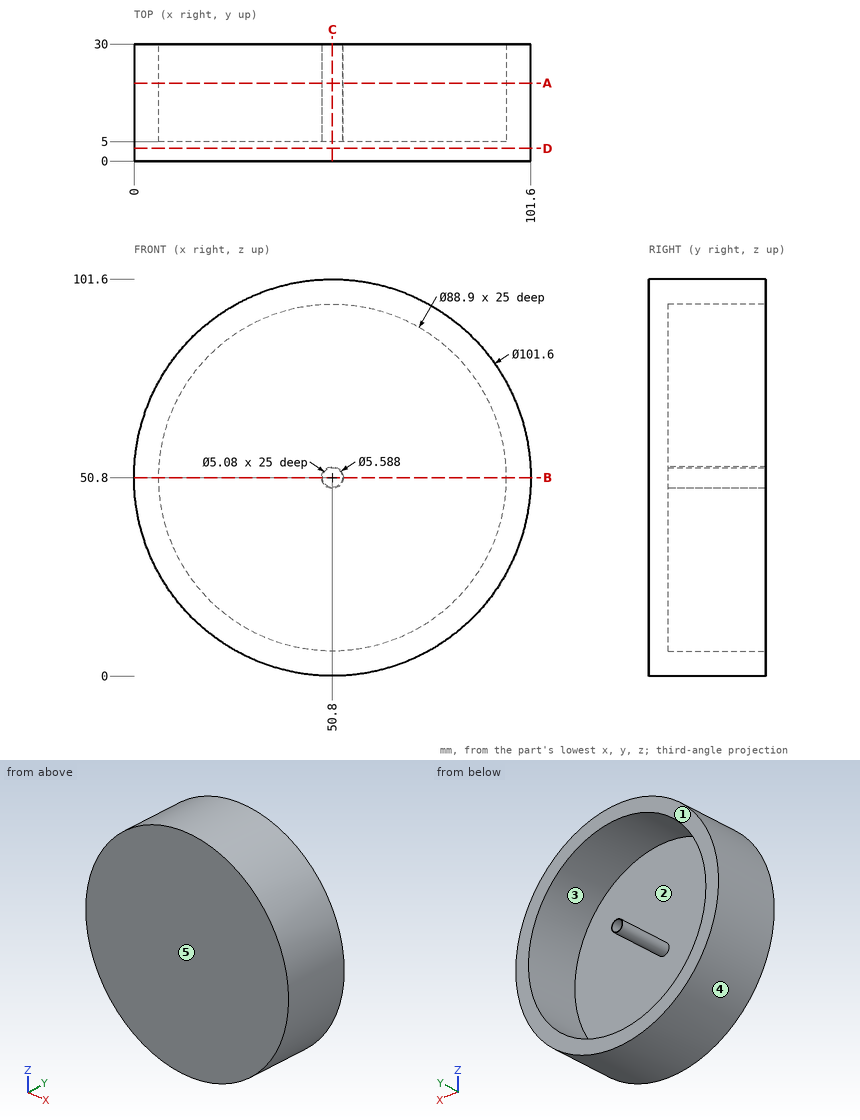
For this review, use the dimensioned drawing (mm, ordinates from the lowest corner) and the shaded views. A direction names the side the tool comes from. Round coordinates to 2 decimals unless told otherwise and drop trailing zeros. Order: outer loops, then holes, each group sorted by start corner. A loop starts at its lowest first (then second) coordinate and runs counter-clockwise, first axis right, second up. Notation, with made-up numbers: (83.25, 61) -> (118.25, 61) arc R19 cw to (118.25, 96) -> close; hole circle Ø8 at (-2, 26.25). An arc over 180 degrees is marked (long way). One line per item, written item: value. Start each with the question number.
Q1. Wall thickness on line 1 (Z direction, x = 50.8, y = 23.5); line 2 (Z direction, x = 55, y = 15.75): over which ranges is each line inside the solid? List them lowest first.
Q2. Mouldability with a two-part tool opening along X and no side actions: class the marked faces 3, 4 and 5 as released by +X, released by -X, zero draft, split by the parting line, or undercut.
Q3. Machinability: for the marked faces 1 and 2, which of the approach directions +Z, -Z, +X, -X, +Y, -Y give a long, thin tool a straight path to every point of the face, cutting with its end or side? Answer none if there is none.
Q4. Take a section at B-B (z = 50.8). Write out the cut boundary in (x, y).
Q5. Take a section at C-C (x = 50.8). Write out the cut boundary in (y, z), and give its area (3 significant figures).
Q6. Take a section at D-D (y = 3.25). Write out the cut boundary in (x, z), and give its area (3 significant figures).
Q7. Clearance check with flat-ended pins moving along their axes: pin 1 Ø6.5 at (x, z) = (50.8, 50.8) entering from +Y; pin 2 Ø1 at (y, z) = (25, 37.5) entering from -X; pin 3 Ø4 at (x, z) = (13.5, 52.5) entering from +Y; pin 4 Ø1 at (y, z) = (22, 18.5) entering from +X. State where each tip first meets the part, or that it passes through.
Q8. Take a section at A-A (y = 20). Write out the cut boundary in (x, z).
Reported:
1. line 1: z = 0 to 6.35, 48.01 to 48.26, 53.34 to 53.59, 95.25 to 101.6
1. line 2: z = 0.17 to 6.55, 95.05 to 101.43
2. face 3: undercut
2. face 4: split by the parting line
2. face 5: zero draft
3. face 1: +Z, -Z, +X, -X, +Y
3. face 2: +Y
4. outline: (0, 0) -> (101.6, 0) -> (101.6, 30) -> (95.25, 30) -> (95.25, 5) -> (53.59, 5) -> (53.59, 30) -> (53.34, 30) -> (53.34, 5) -> (48.26, 5) -> (48.26, 30) -> (48.01, 30) -> (48.01, 5) -> (6.35, 5) -> (6.35, 30) -> (0, 30) -> close
5. outline: (0, 0) -> (30, 0) -> (30, 6.35) -> (5, 6.35) -> (5, 48.01) -> (30, 48.01) -> (30, 48.26) -> (5, 48.26) -> (5, 53.34) -> (30, 53.34) -> (30, 53.59) -> (5, 53.59) -> (5, 95.25) -> (30, 95.25) -> (30, 101.6) -> (0, 101.6) -> close
5. area: 838 mm2
6. outline: circle Ø101.6 at (50.8, 50.8)
6. area: 8,110 mm2
7. pin 1: stops at y = 30
7. pin 2: stops at x = 1.64
7. pin 3: stops at y = 5
7. pin 4: stops at x = 90.42
8. outline: circle Ø101.6 at (50.8, 50.8); circle Ø5.59 at (50.8, 50.8); hole circle Ø88.9 at (50.8, 50.8); hole circle Ø5.08 at (50.8, 50.8)
